```python
from build123d import *

# Parameters (mm, degrees)
SKETCH1_R           = 14.5
BOSS_EXTRUDE1_DEPTH = 1
SKETCH2_R           = 14.5
SKETCH2_R_2         = 12
BOSS_EXTRUDE2_DEPTH = 6
SKETCH3_R           = 13
SKETCH3_R_2         = 12
BOSS_EXTRUDE3_DEPTH = 4
FILLET1_R           = 1


with BuildPart() as part:
    # Sketch1 → Boss-Extrude1 (new body)
    with BuildSketch(Plane(origin=(0, 0, 0), x_dir=(1, 0, 0), z_dir=(0, 1, 0))):
        Circle(SKETCH1_R)
    extrude(amount=BOSS_EXTRUDE1_DEPTH)

    # Sketch2 → Boss-Extrude2 (add)
    with BuildSketch(Plane(origin=(0, 1, 0), x_dir=(1, 0, 0), z_dir=(0, 1, 0))):
        Circle(SKETCH2_R)
        Circle(SKETCH2_R_2, mode=Mode.SUBTRACT)
    extrude(amount=BOSS_EXTRUDE2_DEPTH)

    # Sketch3 → Boss-Extrude3 (add)
    with BuildSketch(Plane(origin=(0, 7, 0), x_dir=(1, 0, 0), z_dir=(0, 1, 0))):
        Circle(SKETCH3_R)
        Circle(SKETCH3_R_2, mode=Mode.SUBTRACT)
    extrude(amount=BOSS_EXTRUDE3_DEPTH)

    # Fillet1
    fillet1_edges = [part.edges().sort_by_distance(p)[0] for p in [
        (-14.5, 0, 0),
    ]]
    fillet(fillet1_edges, radius=FILLET1_R)


solid = part.part
```
Work out the finished part from the listing and answer in its coordinate system (mm). A direction names the side the tool comes from. Round coordinates to 2 decimals unless told otherwise and drop trailing zeros. Loops run counter-clockwise (first coordinate to the right, second up) from the corner with the lowest first, then second, coordinate; pieces in that order, holes last.
(1) For faces 1 (the cylindrical face through (6.691, 3.958, 12.864)), 2 (the flat face through (0, 1, 0)), determine the directions among +Z, -Z, +X, -X, +Y, -Y from which every point of the face is accessible in a straight line to the end or side of a thin tool.
Computed values:
face 1: +Y, -Y
face 2: +Y
(2) Each of these flat-tipped pins is pushed along its axis until it touches: P1, Ø4, axis at y = 6.5, z = 10, coming from the +X side; P2, Ø5, axis at x = 8.5, y = 6, coming from the +Z side; P3, Ø5, axis at x = 2, z = 5.5, coming from the +Y side. Where does it stop, or does it pass through?
Computed values:
P1: stops at x = 12.09
P2: stops at z = 13.2
P3: stops at y = 1
(3) The part is cut by section C-C, the plane y = 7.5. Give the vertices of the cut face in (x, z), and give its area (3 significant figures).
Computed values:
outline: circle Ø26 at (0, 0); hole circle Ø24 at (0, 0)
area: 78.5 mm2
(4) The part is cut by section D-D, the plane y = 1.5. Give the vertices of the cut face in (x, z), and give its area (3 significant figures).
Computed values:
outline: circle Ø29 at (0, 0); hole circle Ø24 at (0, 0)
area: 208 mm2
(5) Find the intervals of material crossed by L1, parallel to X at y = 5, z = 0; L2, parallel to X at y = 9.25, z = 0, in increasing order.
Computed values:
L1: x = -14.5 to -12, 12 to 14.5
L2: x = -13 to -12, 12 to 13
(6) The part is cut by section A-A, the plane z = 0. Give the vertices of the cut face in (x, y), and give its area (3 significant figures).
Computed values:
outline: (-14.5, 1) arc R1 ccw to (-13.5, 0) - (13.5, 0) arc R1 ccw to (14.5, 1) - (14.5, 7) - (13, 7) - (13, 11) - (12, 11) - (12, 1) - (-12, 1) - (-12, 11) - (-13, 11) - (-13, 7) - (-14.5, 7) - close
area: 66.6 mm2
(7) The part is cut by section B-B, the plane x = 0. Give the vertices of the cut face in (y, z).
Computed values:
outline: (0, -13.5) arc R1 ccw to (1, -14.5) - (7, -14.5) - (7, -13) - (11, -13) - (11, -12) - (1, -12) - (1, 12) - (11, 12) - (11, 13) - (7, 13) - (7, 14.5) - (1, 14.5) arc R1 ccw to (0, 13.5) - close
